Part print with two shaded views. Sizes in mm from the minimum x, y, z corner. Coordinates: 2 decimals unless noted, no trailing zeros. Loops run counter-clockwise (first coordinate to the right, second up) from the corner with the lowest first, then second, coordinate; pieces in that order, holes last. Notation, with made-up numbers: (39.5, 45.25) -> (78.5, 45.25) arc R25 cw to (78.5, 60.25) -> close; hole circle Ø10 at (16.5, 49). An arc over 180 degrees is marked (long way). Return JSON: item names as keys, results as strings. Group by question number.
(1) Saw through at D-D on y = 61. Write the cut outline in (x, z).
(2) Saw through at A-A on y = 16.5. Give the number of separate pieces and of enclosed holes in the cut face, then the cut area to 3 significant figures.
(3) Probe L1, parallel to Y at x = 5.5, z = 75.5; L2, parallel to Y at x = 3, z = 48; L3, parallel to Y at x = 5.75, z = 17 (1 decimal). List the from-to ranges inside material, lowest first.
(4) Flat gauge pins, fed straight in: pin 1 Ø5.5 at (y, z) = (18.44, 76.81) entering from -X; pin 2 Ø2 at (x, z) = (3, 29) entering from -Y. Where does each tip first touch, or does it go through?
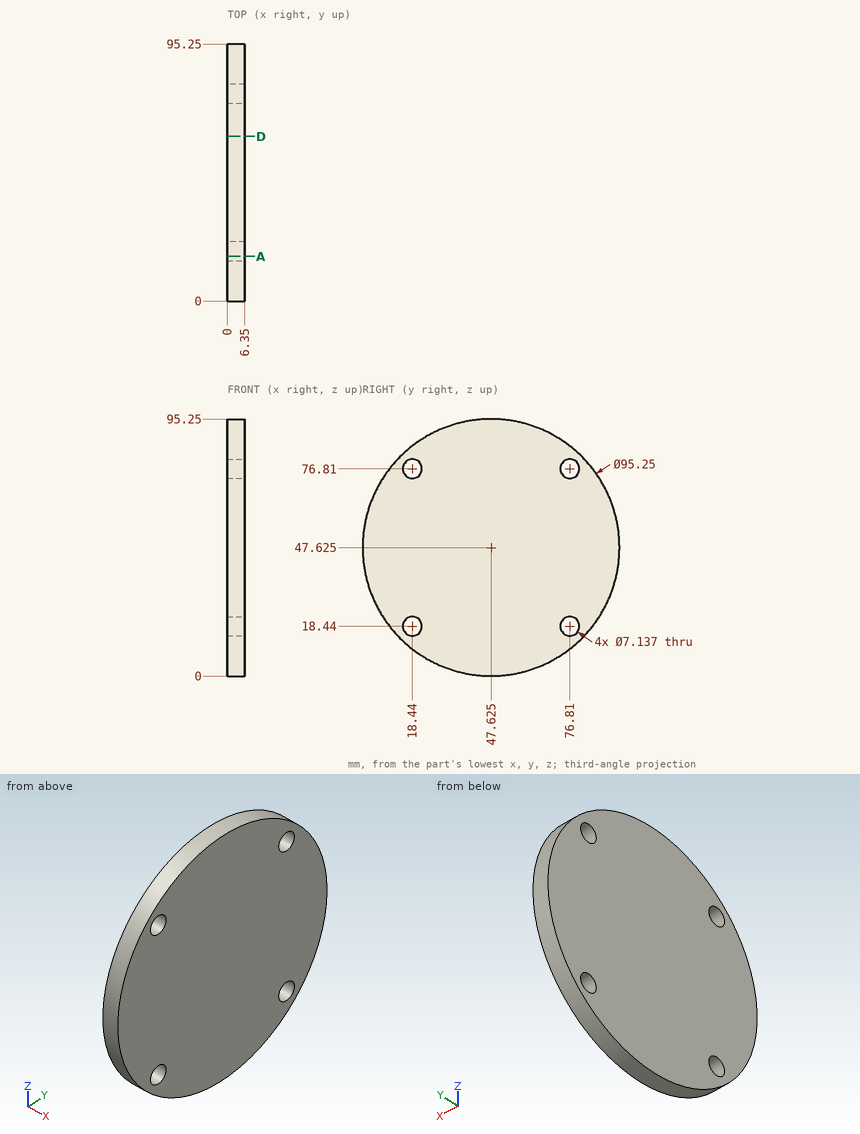
Geometry results:
{
 "1": {"outline": "(0, 1.92) -> (6.35, 1.92) -> (6.35, 93.33) -> (0, 93.33) -> close"},
 "2": {"separate pieces": "3", "enclosed holes": "0", "area": "382 mm²"},
 "3": {"L1": "9.01 to 15.12, 21.76 to 73.49, 80.13 to 86.24", "L2": "0 to 95.25", "L3": "11.2 to 15.2, 21.7 to 73.5, 80.1 to 84.1"},
 "4": {"pin 1": "through", "pin 2": "y = 3.38"}
}
